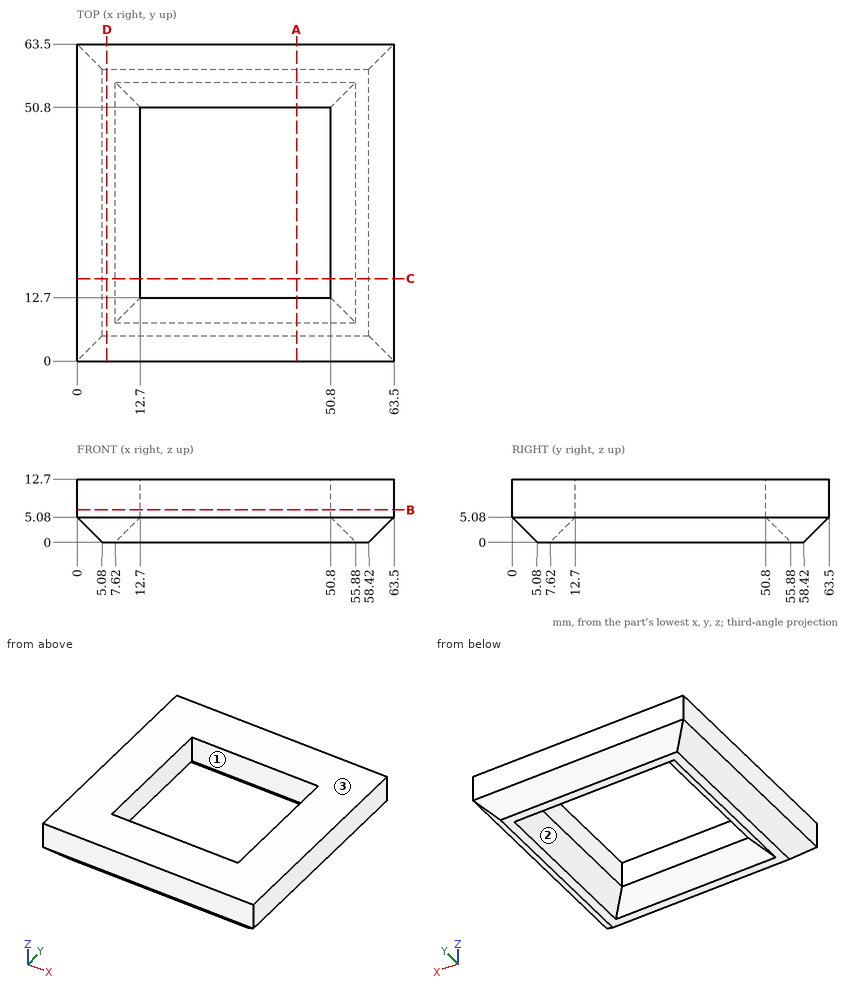
Input: dimensioned drawing with shaded views. Units: mm. Origin: part minimum x, y, z. A direction names the side the tool comes from. Coordinates: 2 decimals unless noted, no trailing zeros. Order: outer loops, then holes, each group sorted by start corner. A loop starts at its lowest first (then second) coordinate and runs counter-clockwise, first axis right, second up.
(1) Section query D-D (x = 6). Return the cut outline in (y, z), plus the area to 3 significant figures.
(2) Access query for the marked faces 1, 2 and 3. Directions: +Z, -Z, +X, -X, +Y, -Y. A direction counts if a zero-diameter tool reaches every point of the face in a straight line with its end or side. Return the directions, or none.
(3) First-contact query: pin 1 (4 mm diameter, centred on x = 23.5, z = 2.5, fed in from -Y); pin 2 (1.5 mm diameter, centred on x = 15, z = 4, fed in from -Y); pin 3 (1.5 mm diameter, centred on x = 44, z = 2, fed in from -Y). Flat tips, straight axial feed; report the tip coordinate or a pass-through.
(4) Section query A-A (x = 44). Return the cut outline in (y, z), plus the area to 3 significant figures.
(5) Material intervals for probe 1 along Y at (x, z) = (18, 6.75); probe 2 along X at (y, z) = (29, 3.75), sorted ascending.
(6) Section query B-B (z = 6.5). Return the cut outline in (x, y).
Solution:
1. outline: (0, 5.08) - (5.08, 0) - (58.42, 0) - (63.5, 5.08) - (63.5, 12.7) - (0, 12.7) - close
1. area: 781 mm2
2. face 1: +Z, -Z
2. face 2: -Z
2. face 3: +Z, +X, -X, +Y, -Y
3. pin 1: stops at y = 0.58
3. pin 2: stops at y = 0.33
3. pin 3: stops at y = 2.33
4. outline: (0, 5.08) - (5.08, 0) - (7.62, 0) - (12.7, 5.08) - (12.7, 12.7) - (0, 12.7) - close; (50.8, 5.08) - (55.88, 0) - (58.42, 0) - (63.5, 5.08) - (63.5, 12.7) - (50.8, 12.7) - close
4. area: 271 mm2
5. probe 1: y = 0 to 12.7, 50.8 to 63.5
5. probe 2: x = 1.33 to 11.37, 52.13 to 62.17
6. outline: (0, 0) - (63.5, 0) - (63.5, 63.5) - (0, 63.5) - close; hole (12.7, 12.7) - (50.8, 12.7) - (50.8, 50.8) - (12.7, 50.8) - close
